from build123d import *

# Parameters (mm, degrees)
SKETCH1_W           = 88.9
SKETCH1_H           = 50.8
BOSS_EXTRUDE1_DEPTH = 5.588
CUT_EXTRUDE1_REACH  = 53.499
SKETCH2_R           = 1.778
SKETCH2_R_2         = 1.5
FILLET1_R           = 2.54
CHAMFER1_SIZE       = 1.65


with BuildPart() as part:
    # Sketch1 → Boss-Extrude1 (new body)
    with BuildSketch(Plane(origin=(0, 0, 0), x_dir=(1, 0, 0), z_dir=(0, 1, 0))):
        Rectangle(SKETCH1_W, SKETCH1_H)
    extrude(amount=BOSS_EXTRUDE1_DEPTH)

    # Sketch2 → Cut-Extrude1 (cut, up to next)
    with BuildSketch(Plane(origin=(0, 5.588, 0), x_dir=(1, 0, 0), z_dir=(0, 1, 0)), mode=Mode.PRIVATE) as cut_extrude1_sk1:
        with Locations(Location((-38.1, -9.779, 0), (0, 0, 270))):
            Circle(SKETCH2_R)
    cut_extrude1_tool1 = extrude(cut_extrude1_sk1.sketch, amount=-CUT_EXTRUDE1_REACH, mode=Mode.PRIVATE) & part.part
    # Sketch2 → Cut-Extrude1 (cut, up to next)
    with BuildSketch(Plane(origin=(0, 5.588, 0), x_dir=(1, 0, 0), z_dir=(0, 1, 0)), mode=Mode.PRIVATE) as cut_extrude1_sk2:
        with Locations(Location((-38.1, 9.779, 0), (0, 0, 270))):
            Circle(SKETCH2_R)
    cut_extrude1_tool2 = extrude(cut_extrude1_sk2.sketch, amount=-CUT_EXTRUDE1_REACH, mode=Mode.PRIVATE) & part.part
    # Sketch2 → Cut-Extrude1 (cut, up to next)
    with BuildSketch(Plane(origin=(0, 5.588, 0), x_dir=(1, 0, 0), z_dir=(0, 1, 0)), mode=Mode.PRIVATE) as cut_extrude1_sk3:
        with Locations(Location((-19.05, -15.875, 0), (0, 0, 270))):
            Circle(SKETCH2_R_2)
    cut_extrude1_tool3 = extrude(cut_extrude1_sk3.sketch, amount=-CUT_EXTRUDE1_REACH, mode=Mode.PRIVATE) & part.part
    # Sketch2 → Cut-Extrude1 (cut, up to next)
    with BuildSketch(Plane(origin=(0, 5.588, 0), x_dir=(1, 0, 0), z_dir=(0, 1, 0)), mode=Mode.PRIVATE) as cut_extrude1_sk4:
        with Locations(Location((-19.05, 15.875, 0), (0, 0, 270))):
            Circle(SKETCH2_R_2)
    cut_extrude1_tool4 = extrude(cut_extrude1_sk4.sketch, amount=-CUT_EXTRUDE1_REACH, mode=Mode.PRIVATE) & part.part
    cut_extrude1_1 = cut_extrude1_tool1.solids().sort_by_distance((-38.1, 5.588, 9.779))[0]
    add(cut_extrude1_1, mode=Mode.SUBTRACT)
    cut_extrude1_2 = cut_extrude1_tool2.solids().sort_by_distance((-38.1, 5.588, -9.779))[0]
    add(cut_extrude1_2, mode=Mode.SUBTRACT)
    cut_extrude1_3 = cut_extrude1_tool3.solids().sort_by_distance((-19.05, 5.588, 15.875))[0]
    add(cut_extrude1_3, mode=Mode.SUBTRACT)
    cut_extrude1_4 = cut_extrude1_tool4.solids().sort_by_distance((-19.05, 5.588, -15.875))[0]
    add(cut_extrude1_4, mode=Mode.SUBTRACT)
    cut_extrude1 = cut_extrude1_1 + cut_extrude1_2 + cut_extrude1_3 + cut_extrude1_4  # Cut-Extrude1 as one shape, for the pattern or mirror that repeats it

    # Mirror1: Cut-Extrude1 across plane
    add(cut_extrude1.mirror(Plane(origin=(0, 0, 0), x_dir=(0, 0, 1), z_dir=(1, 0, 0))), mode=Mode.SUBTRACT)

    # Fillet1
    fillet1_edges = [part.edges().sort_by_distance(p)[0] for p in [
        (44.45, 2.794, 25.4),
        (-44.45, 2.794, 25.4),
        (-44.45, 2.794, -25.4),
        (44.45, 2.794, -25.4),
    ]]
    fillet(fillet1_edges, radius=FILLET1_R)

    # Chamfer1
    chamfer1_edges = [part.edges().sort_by_distance(p)[0] for p in [
        (-19.05, 5.588, -17.375),
        (-19.05, 5.588, 14.375),
        (19.05, 5.588, -17.375),
        (19.05, 5.588, 14.375),
    ]]
    chamfer(chamfer1_edges, length=CHAMFER1_SIZE)


solid = part.part
Verification items for the finished model (mm, model axes). Round coordinates to 2 decimals unless told otherwise and drop trailing zeros. Loops run counter-clockwise (first coordinate to the right, second up) from the corner with the lowest first, then second, coordinate; pieces in that order, holes last. Notation, with made-up numbers: (-31, 76) - (-3, 76) arc R15 ccw to (-3, 80) - close; hole circle Ø5 at (-19, 64.5). An arc over 180 degrees is marked (long way). Use one line per item in the form item = value.
1. Section check B-B on y = 0.9. Give the number of separate pieces and of enclosed holes in the cut face, and give its area (3 significant figures).
A:
separate_pieces = 1
enclosed_holes = 8
area = 4,440 mm²
2. Section check A-A on x = -38.1. Record the cut outline in (y, z), and give its area (3 significant figures).
A:
outline = (0, -25.4) - (5.59, -25.4) - (5.59, -11.56) - (0, -11.56) - close; (0, -8) - (5.59, -8) - (5.59, 8) - (0, 8) - close; (0, 11.56) - (5.59, 11.56) - (5.59, 25.4) - (0, 25.4) - close
area = 244 mm²
3. Gauge pin test, flat ends, axial feed: pin 1 Ø3.5 at (x, z) = (19.05, -15.875) entering from -Y; pin 2 Ø5 at (x, z) = (19.05, 15.875) entering from +Y. Record the tip position at first contact, or that the pin passes through.
A:
pin_1 = 0
pin_2 = 4.94
4. Scan lines: probe 1 along Z at (x, y) = (38.1, 2.5); probe 2 along Z at (x, y) = (19.05, 1.25) (3 decimals); probe 3 along X at (y, z) = (2, 10). Record each from-to range of solid material in increasing order.
A:
probe_1 = -25.4 to -11.56, -8 to 8, 11.56 to 25.4
probe_2 = -25.4 to -17.375, -14.375 to 14.375, 17.375 to 25.4
probe_3 = -44.45 to -39.86, -36.34 to 36.34, 39.86 to 44.45
5. Section check C-C on x = 19.05. Record the cut outline in (y, z) (3 decimals).
A:
outline = (0, -25.4) - (5.588, -25.4) - (5.588, -19.025) - (3.938, -17.375) - (0, -17.375) - close; (0, -14.375) - (3.938, -14.375) - (5.588, -12.725) - (5.588, 12.725) - (3.938, 14.375) - (0, 14.375) - close; (0, 17.375) - (3.938, 17.375) - (5.588, 19.025) - (5.588, 25.4) - (0, 25.4) - close
